Verification items for the finished model (mm, model axes). Coordinates: 2 decimals unless noted, no trailing zeros. Write each loop counter-clockwise with the first axis right and the second up, starting at its lowest first coordinate (ties: lowest second). Pieces come first, ordered by that corner, then holes. Notation, with made-up numbers: (36.25, 52.25) - (74.25, 52.25) arc R36 cw to (74.25, 90.25) - close; hole circle Ø5 at (83, -8). An arc over 180 degrees is marked (long way). Use one line per item in the form item = value. Start each with the question number.
(1) Sectioned sample at A-A (x = -13.5). Record the cut outline in (y, z).
(2) Gauge pin test, flat end, axial feed: pin 1 Ø1 at (x, z) = (-3, 2.5) entering from -Y. Record the tip position at first contact, or that the pin passes through.
(3) Sectioned sample at D-D (y = 1.25). Record the cut outline in (x, z), and give its area (3 significant figures).
(4) Sectioned sample at C-C (y = 4). Record the cut outline in (x, z).
(5) Material ranges on line 1 (Y direction, x = -5.25, z = 3.9); line 2 (X direction, y = 7.5, z = 1.95); line 3 (X direction, y = 7.75, z = 0.6), recorded low to high. Write a range as [from, to].
(6) Sectioned sample at B-B (z = 3.75). Record the cut outline in (x, y).
from build123d import *

# Parameters (mm, degrees)
SALIENTE_EXTRUIR1_DEPTH = 5
REDONDEO1_R             = 1


with BuildPart() as part:
    # Croquis1 → Saliente-Extruir1 (new body)
    with BuildSketch(Plane.XY):
        Polygon((0, 8), (0, 0), (-15, 5.459553514), (-15, 8), align=None)
    extrude(amount=SALIENTE_EXTRUIR1_DEPTH)

    # Redondeo1
    redondeo1_edges = [part.edges().sort_by_distance(p)[0] for p in [
        (-7.5, 8, 0),
        (-15, 8, 2.5),
        (0, 8, 2.5),
        (-7.5, 8, 5),
    ]]
    fillet(redondeo1_edges, radius=REDONDEO1_R)


solid = part.part
Answers below:
q1.outline = (4.91, 0) - (7, 0) arc R1 ccw to (8, 1) - (8, 4) arc R1 ccw to (7, 5) - (4.91, 5) - close
q2.pin_1 = 0.91
q3.outline = (-3.43, 0) - (0, 0) - (0, 5) - (-3.43, 5) - close
q3.area = 17.2 mm2
q4.outline = (-10.99, 0) - (0, 0) - (0, 5) - (-10.99, 5) - close
q5.line_1 = [1.91, 8]
q5.line_2 = [-14.87, -0.13]
q5.line_3 = [-14.66, -0.34]
q6.outline = (-15, 5.46) - (0, 0) - (0, 7) arc R1 ccw to (-1, 8) - (-14, 8) arc R1 ccw to (-15, 7) - close
